The figure shows three views and two pictorial views of one solid part (mm, origin at its lowest corner). Answer the questions. Give positions to 0.01 mm unless a question says otherwise; leave off trailing zeros. Loops run counter-clockwise (first coordinate to the right, second up) from the corner with the lowest first, then second, coordinate; pieces in that order, holes last. Notation, with made-up numbers: M -8,70.5 L 39,70.5 A31 cw 39,96.5 Z; hole C 34,-3 d5. An arc over 180 degrees is marked long. One line per item, written item: value. Start each with the question number.
Q1. A cutting plane is placed at B-B, the plane z = 117. Determine the outline of the cut face in (x, y), and give its area (3 significant figures).
Q2. A cutting plane is placed at A-A, the plane x = 11. Determine the outline of the cut face in (y, z), and give its area (3 significant figures).
Q3. Consider L1, parallel to Y at x = 17.5, z = 195. Determine where the line is inside the solid, lowest interval first.
Q4. Flat-ended cylindrical pins translate along their axes: pin 1 (5.5 mm diameter, centred on x = 13, y = 481.5, fed in from -Z); pin 2 (9.5 mm diameter, centred on x = 6, z = 156.5, fed in from -Y); pin 3 (5.5 mm diameter, centred on x = 10.5, y = 484.5, fed in from +Z). Find the tip coordinate at first contact, or state that the pin passes through.
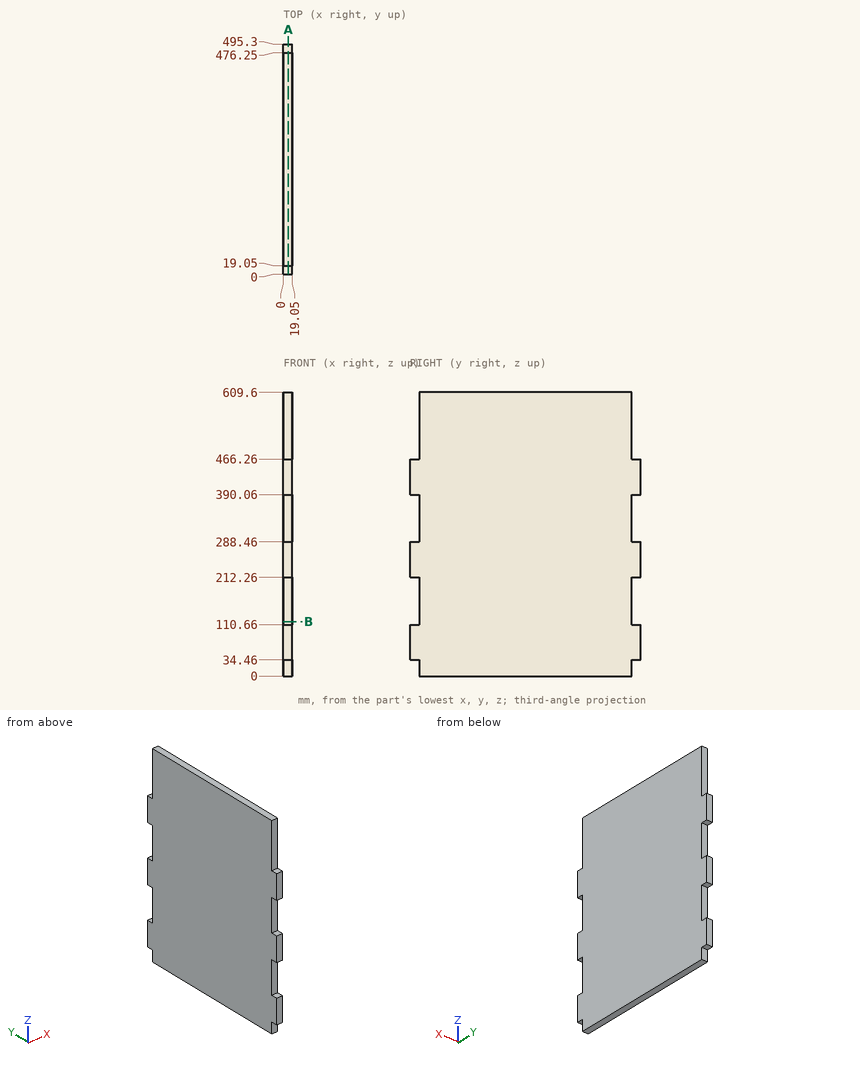
Answer block:
1. outline: M 0,19.05 L 19.05,19.05 L 19.05,476.25 L 0,476.25 Z
1. area: 8,710 mm^2
2. outline: M 0,34.46 L 19.05,34.46 L 19.05,0 L 476.25,0 L 476.25,34.46 L 495.3,34.46 L 495.3,110.66 L 476.25,110.66 L 476.25,212.26 L 495.3,212.26 L 495.3,288.46 L 476.25,288.46 L 476.25,390.06 L 495.3,390.06 L 495.3,466.26 L 476.25,466.26 L 476.25,609.6 L 19.05,609.6 L 19.05,466.26 L 0,466.26 L 0,390.06 L 19.05,390.06 L 19.05,288.46 L 0,288.46 L 0,212.26 L 19.05,212.26 L 19.05,110.66 L 0,110.66 Z
2. area: 287,000 mm^2
3. L1: 19.05 to 476.25
4. pin 1: z = 34.46
4. pin 2: y = 19.05
4. pin 3: z = 466.26
